Part model, mm, in its own coordinate system. A direction names the side the tool comes from. Coordinates: 2 decimals unless noted, no trailing zeros. Write each loop counter-clockwise with the first axis right and the second up, starting at its lowest first coordinate (ties: lowest second). Pieces come first, ordered by that corner, then holes. Notation, with made-up numbers: M 15,-10.75 L 74,-10.75 A19 ccw 74,24.25 Z; hole C -25,62 d5. An arc over 180 degrees is marked long. Use a Markdown table: item, result. Add a question column.
Q1. Slice it at A-A on z = 3.5. Write the cut outline in (x, y), then the cut area to 3 significant figures.
Q2. Wall check: L1, parallel to Y at x = 90, z = 1.45; L2, parallel to X at y = 2, z = 5.75; L3, parallel to Y at x = 90, z = 5.55. Give the ranges that are in metal, low to high. Write a range as from..to.
Q3. Tool access for faces 1 (the cylindrical face through (94, -3, 2)), 2 (the flat face through (90, -8, 4.5)): list every direction of +Z, -Z, +X, -X, +Y, -Y with a clear straight run to the whole face (end or side of a thin tool).
Q4. Pin check, flat tips, straight feed: pin 1 Ø4 at (x, y) = (90, 4) entering from +Z; pin 2 Ø1.9 at (x, y) = (90, -10) entering from -Z; pin 3 Ø1 at (y, z) = (-5, 5.5) entering from -X; pin 4 Ø1 at (y, z) = (5.5, 5.5) entering from +X. Stop position of each tip, or through.
Q5. Slice it at C-C on x = 97. Write the cut outline in (y, z), then the cut area to 3 significant figures.
Q6. Slice it at D-D on x = 42. Write the cut outline in (y, z), then the cut area to 3 significant figures.
Q7. Slice it at B-B on y = -3. Write the cut outline in (x, z), then the cut area to 3 significant figures.
from build123d import *

# Parameters (mm, degrees)
EXTRUDE_1_DEPTH     = 7
SKETCH_2_R          = 4.1
SKETCH_2_R_2        = 1.6
SKETCH_2_R_3        = 4
CUT_EXTRUDE_1_DEPTH = 10
SKETCH_3_R          = 11
CUT_EXTRUDE_2_DEPTH = 2.5


with BuildPart() as part:
    # 草图1 → 凸台-拉伸1 (new body)
    with BuildSketch(Plane.XY):
        with BuildLine():
            Line((0, -10), (90, -18))
            ThreePointArc((90, -18), (105, -3), (90, 12))
            Line((90, 12), (0, 10))
            ThreePointArc((0, 10), (-10, 0), (0, -10))
        make_face()
    extrude(amount=EXTRUDE_1_DEPTH)

    # 草图2 → 切除-拉伸1 (cut)
    with BuildSketch(Plane(origin=(0, 0, 0), x_dir=(-1, 0, 0), z_dir=(0, 0, -1))):
        Circle(SKETCH_2_R)
        with Locations((-90, -10)):
            Circle(SKETCH_2_R_2)
        with Locations((-83, -3)):
            Circle(SKETCH_2_R_2)
        with Locations((-90, 4)):
            Circle(SKETCH_2_R_2)
        with Locations((-97, -3)):
            Circle(SKETCH_2_R_2)
        with Locations((-90, -3)):
            Circle(SKETCH_2_R_3)
    extrude(amount=-CUT_EXTRUDE_1_DEPTH, mode=Mode.SUBTRACT)

    # 草图3 → 切除-拉伸2 (cut)
    with BuildSketch(Plane.XY.offset(7)):
        with Locations((90, -3)):
            Circle(SKETCH_3_R)
    extrude(amount=-CUT_EXTRUDE_2_DEPTH, mode=Mode.SUBTRACT)


solid = part.part
Recorded:
| question | item | result |
|---|---|---|
| 1 | outline | M 0,-10 L 90,-18 A15 ccw 90,12 L 0,10 A10 ccw Z; hole C 0,0 d8.2; hole C 83,-3 d3.2; hole C 90,-3 d8; hole C 90,-10 d3.2; hole C 90,4 d3.2; hole C 97,-3 d3.2 |
| 1 | area | 2,630 mm² |
| 2 | L1 | -18..-11.6, -8.4..-7, 1..2.4, 5.6..12 |
| 2 | L2 | -9.8..-3.58, 3.58..80.2, 99.8..104.14 |
| 2 | L3 | -18..-14, 8..12 |
| 3 | face 1 | +Z, -Z |
| 3 | face 2 | +Z |
| 4 | pin 1 | z = 4.5 |
| 4 | pin 2 | through |
| 4 | pin 3 | x = -8.93 |
| 4 | pin 4 | x = 102.69 |
| 5 | outline | M -16.27,0 L -4.6,0 L -4.6,4.5 L -11.49,4.5 L -11.49,7 L -16.27,7 Z; M -1.4,0 L 10.27,0 L 10.27,7 L 5.49,7 L 5.49,4.5 L -1.4,4.5 Z |
| 5 | area | 129 mm² |
| 6 | outline | M -13.73,0 L 10.93,0 L 10.93,7 L -13.73,7 Z |
| 6 | area | 173 mm² |
| 7 | outline | M -9.54,0 L -2.79,0 L -2.79,7 L -9.54,7 Z; M 2.79,0 L 81.4,0 L 81.4,4.5 L 79,4.5 L 79,7 L 2.79,7 Z; M 84.6,0 L 86,0 L 86,4.5 L 84.6,4.5 Z; M 94,0 L 95.4,0 L 95.4,4.5 L 94,4.5 Z; M 98.6,0 L 105,0 L 105,7 L 101,7 L 101,4.5 L 98.6,4.5 Z |
| 7 | area | 643 mm² |
